from build123d import *

# Parameters (mm, degrees)
SWEEP1_PROFILE_R     = 11
CUT_SWEEP1_PROFILE_R = 7.5
SKETCH34_R           = 10
SKETCH34_R_2         = 7.5
BOSS_EXTRUDE1_DEPTH  = 5


with BuildPart() as part:
    # Sweep1: sweep along a path in Sketch1
    with BuildLine(Plane(origin=(0, 0, 0), x_dir=(0, 0, -1), z_dir=(1, 0, 0))) as sweep1_path:
        Line((0, 0), (0, -15))
        ThreePointArc((0, -15), (-4.393398282, -25.606601718), (-15, -30))
        Line((-15, -30), (-30, -30))
    # Sweep1 profile (on start of the path) → Sweep1 (sweep)
    with BuildSketch(Plane(origin=(0, 0, 0), x_dir=(0, 0, -1), z_dir=(0, -1, 0))):
        Circle(SWEEP1_PROFILE_R)
    sweep(path=sweep1_path.line)

    # Cut-Sweep1: sweep along a path in Sketch1_2
    with BuildLine(Plane(origin=(0, 0, 0), x_dir=(0, 0, -1), z_dir=(1, 0, 0))) as cut_sweep1_path:
        Line((0, 0), (0, -15))
        ThreePointArc((0, -15), (-4.393398282, -25.606601718), (-15, -30))
        Line((-15, -30), (-30, -30))
    # Cut-Sweep1 profile (on start of the path) → Cut-Sweep1 (sweep, cut)
    with BuildSketch(Plane(origin=(0, 0, 0), x_dir=(0, 0, -1), z_dir=(0, -1, 0))):
        Circle(CUT_SWEEP1_PROFILE_R)
    sweep(path=cut_sweep1_path.line, mode=Mode.SUBTRACT)

    # Sketch34 → Boss-Extrude1 (add)
    with BuildSketch(Plane(origin=(0, 0, 0), x_dir=(1, 0, 0), z_dir=(0, 1, 0))):
        with Locations(Location((0, 0, 0), (0, 0, 270))):
            Circle(SKETCH34_R)
        with Locations(Location((0, 0, 0), (0, 0, 90))):
            Circle(SKETCH34_R_2, mode=Mode.SUBTRACT)
    extrude(amount=BOSS_EXTRUDE1_DEPTH)


solid = part.part
Geometry check sheet. Reference: the model listing, model coordinates, mm. A direction names the side the tool comes from. Round coordinates to 2 decimals unless told otherwise and drop trailing zeros. Order: outer loops, then holes, each group sorted by start corner. A loop starts at its lowest first (then second) coordinate and runs counter-clockwise, first axis right, second up. Notation, with made-up numbers: (69.5, 5.5) -> (101.5, 5.5) arc R27 cw to (101.5, 38.5) -> close; hole circle Ø7 at (-15, 3). An arc over 180 degrees is marked (long way). Use one line per item in the form item = value.
1. Cross-section at B-B, the plane y = -12. Enter the section's corners in (x, z), plus the area to 3 significant figures.
Working result:
outline = circle Ø22 at (0, 0); hole circle Ø15 at (0, 0)
area = 203 mm^2
2. Set-up check for faces 1 (the face through (7, 5, 4)), 2 (the face through (0.33, -22.507, 22.605)), 3 (the face through (-10.74, -7.6, 2.38)): record each of +Z, -Z, +X, -X, +Y, -Y from which the full face is reachable in a straight line by a thin tool's end or side.
Working result:
face_1 = +Z, -Z, +X, -X, +Y
face_2 = +Z
face_3 = +Y
3. Cross-section at A-A, the plane x = 4. Enter the section's corners in (y, z).
Working result:
outline = (-40.25, 15) arc R25.25 ccw to (-15, -10.25) -> (0, -10.25) -> (0, -9.17) -> (5, -9.17) -> (5, -6.34) -> (-15, -6.34) arc R21.34 cw to (-36.34, 15) -> (-36.34, 30) -> (-40.25, 30) -> close; (-23.66, 15) arc R8.66 ccw to (-15, 6.34) -> (5, 6.34) -> (5, 9.17) -> (0, 9.17) -> (0, 10.25) -> (-15, 10.25) arc R4.75 cw to (-19.75, 15) -> (-19.75, 30) -> (-23.66, 30) -> close
4. Cross-section at D-D, the plane x = -3.5. Enter the section's corners in (y, z).
Working result:
outline = (-40.43, 15) arc R25.43 ccw to (-15, -10.43) -> (0, -10.43) -> (0, -9.37) -> (5, -9.37) -> (5, -6.63) -> (-15, -6.63) arc R21.63 cw to (-36.63, 15) -> (-36.63, 30) -> (-40.43, 30) -> close; (-23.37, 15) arc R8.37 ccw to (-15, 6.63) -> (5, 6.63) -> (5, 9.37) -> (0, 9.37) -> (0, 10.43) -> (-15, 10.43) arc R4.57 cw to (-19.57, 15) -> (-19.57, 30) -> (-23.37, 30) -> close
5. Scan lines: line 1 along Y through (x, z) = (0, 22.25); line 2 along X through (y, z) = (-6, 0); line 3 along X through (y, z) = (-24, 19). Record each from-to range of solid material in increasing order. Write a range as from..to.
Working result:
line_1 = -41..-37.5, -22.5..-19
line_2 = -11..-7.5, 7.5..11
line_3 = -9.22..-4.5, 4.5..9.22
6. Mould release check, pull along X, two halves, no side actions. Record for faces 4 (the face through (-0.33, -5.14, 7.493)), 5 (the face through (-4.213, -40.161, 22.605)), 6 (the face through (-10, 0, -2)): pulls with the +X half, pulls with the -X half, needs draft (parallel to the pull), parting line crosses it, or undercut.
Working result:
face_4 = undercut
face_5 = parting line crosses it
face_6 = needs draft
7. Go/stop test with flat-tipped pins: pin 1 (1.5 mm diameter, centred on x = -7, z = 12.5, fed in from -Y); pin 2 (10 mm diameter, centred on y = -9, z = 7, fed in from -X); pin 3 (3 mm diameter, centred on x = 3, y = -12.5, fed in from +Z). Record where each tip stops, or that it passes through.
Working result:
pin_1 = -38.93
pin_2 = -10.82
pin_3 = 10.9
8. Cross-section at C-C, the plane z = 20.5. Enter the section's corners in (x, y).
Working result:
outline = circle Ø22 at (0, -30); hole circle Ø15 at (0, -30)
